from build123d import *

# Parameters (mm, degrees)
ESBO_O1_W                = 174
ESBO_O1_H                = 124
ESBO_O1_R                = 1.5
RESSALTO_EXTRUS_O1_DEPTH = 2
ESBO_O2_R                = 1.3
ESBO_O2_W                = 20
ESBO_O2_H                = 44
ESBO_O2_W_2              = 27
ESBO_O2_H_2              = 11
CORTE_EXTRUS_O1_DEPTH    = 2


with BuildPart() as part:
    # Esboço1 → Ressalto-extrusão1 (new body)
    with BuildSketch(Plane(origin=(0, 0, 0), x_dir=(1, 0, 0), z_dir=(0, 1, 0))):
        Rectangle(ESBO_O1_W, ESBO_O1_H)
        with Locations(Location((-77, 52, 0), (0, 0, 270))):
            Circle(ESBO_O1_R, mode=Mode.SUBTRACT)
        with Locations(Location((-77, -52, 0), (0, 0, 270))):
            Circle(ESBO_O1_R, mode=Mode.SUBTRACT)
        with Locations(Location((77, -52, 0), (0, 0, 270))):
            Circle(ESBO_O1_R, mode=Mode.SUBTRACT)
        with Locations(Location((77, 52, 0), (0, 0, 270))):
            Circle(ESBO_O1_R, mode=Mode.SUBTRACT)
    extrude(amount=RESSALTO_EXTRUS_O1_DEPTH)

    # Esboço2 → Corte-extrusão1 (cut)
    with BuildSketch(Plane(origin=(0, 2, 0), x_dir=(1, 0, 0), z_dir=(0, 1, 0))):
        with Locations(Location((-13.5, -21, 0), (0, 0, 270))):
            Circle(ESBO_O2_R)
        with Locations(Location((-13.5, -29, 0), (0, 0, 270))):
            Circle(ESBO_O2_R)
        with Locations(Location((-13.5, -37, 0), (0, 0, 270))):
            Circle(ESBO_O2_R)
        with Locations(Location((-13.5, -45, 0), (0, 0, 270))):
            Circle(ESBO_O2_R)
        with Locations(Location((13.5, -37, 0), (0, 0, 90))):
            Circle(ESBO_O2_R)
        with Locations(Location((13.5, -45, 0), (0, 0, 90))):
            Circle(ESBO_O2_R)
        with Locations(Location((13.5, -29, 0), (0, 0, 90))):
            Circle(ESBO_O2_R)
        with Locations(Location((13.5, -21, 0), (0, 0, 90))):
            Circle(ESBO_O2_R)
        with Locations((0, -25)):
            Rectangle(ESBO_O2_W, ESBO_O2_H)
        with BuildLine():
            Line((-37, 45), (-37, -45))
            ThreePointArc((-37, -45), (-42, -50), (-47, -45))
            Line((-47, -45), (-47, 45))
            ThreePointArc((-47, 45), (-42, 50), (-37, 45))
        make_face()
        with BuildLine():
            Line((-57, 45), (-57, -45))
            ThreePointArc((-57, -45), (-62, -50), (-67, -45))
            Line((-67, -45), (-67, 45))
            ThreePointArc((-67, 45), (-62, 50), (-57, 45))
        make_face()
        with BuildLine():
            Line((47, 45), (47, -45))
            ThreePointArc((47, -45), (42, -50), (37, -45))
            Line((37, -45), (37, 45))
            ThreePointArc((37, 45), (42, 50), (47, 45))
        make_face()
        with BuildLine():
            Line((67, 45), (67, -45))
            ThreePointArc((67, -45), (62, -50), (57, -45))
            Line((57, -45), (57, 45))
            ThreePointArc((57, 45), (62, 50), (67, 45))
        make_face()
        with BuildLine():
            Line((-20.724176636, 23), (20.724176636, 23))
            ThreePointArc((20.724176636, 23), (25.724176636, 18), (20.724176636, 13))
            Line((20.724176636, 13), (-20.724176636, 13))
            ThreePointArc((-20.724176636, 13), (-25.724176636, 18), (-20.724176636, 23))
        make_face()
        with Locations((0, 46.5)):
            Rectangle(ESBO_O2_W_2, ESBO_O2_H_2)
    extrude(amount=-CORTE_EXTRUS_O1_DEPTH, mode=Mode.SUBTRACT)


solid = part.part
The model under review builds one solid part; all positions refer to its coordinate system, in mm. A direction names the side the tool comes from. Coordinates: 2 decimals unless noted, no trailing zeros. Loops run counter-clockwise (first coordinate to the right, second up) from the corner with the lowest first, then second, coordinate; pieces in that order, holes last. Notation, with made-up numbers: (-26, 32.5) -> (-21, 32.5) arc R36 ccw to (-21, 69.5) -> close; hole circle Ø5 at (-6.75, 78). An arc over 180 degrees is marked (long way). Use a Markdown table: item, result. Add a question column.
1. Draft analysis for pull direction X (two halves, no side actions). For faces 3 (the face through (62, 1, 50)), 4 (the face through (-1, 2, -1)), 5 (the face through (42, 1, -50)), state which applies: pulls with the +X half, pulls with the -X half, needs draft (parallel to the pull), parting line crosses it, or undercut.
2. Add section C-C on z = 41. Write out the cut boundary in (x, y), plus the area to 3 significant figures.
3. Add section B-B on x = 1. Write out the cut boundary in (y, z).
4. Add section A-A on z = -33. Write out the cut boundary in (x, y), plus the area to 3 significant figures.
5. Machinability: for faces 1 (the face through (-1, 0, -1)), 2 (the face through (42, 1, 50)), which of the approach directions +Z, -Z, +X, -X, +Y, -Y give a long, thin tool a straight path to every point of the face, cutting with its end or side? Answer none if there is none.
6. Add section D-D on x = 39.5. Write out the cut boundary in (y, z).
7. To check wall thickness, follow line 1 (X direction, y = 1.2, z = -25); line 2 (Z direction, x = 5, y = 0.5); line 3 (X direction, y = 0.5, z = 52). State the ranges of each line that lie inside material, in increasing order.
Returned:
| question | item | result |
|---|---|---|
| 1 | face 3 | undercut |
| 1 | face 4 | needs draft |
| 1 | face 5 | undercut |
| 2 | outline | (-87, 0) -> (-67, 0) -> (-67, 2) -> (-87, 2) -> close; (-57, 0) -> (-47, 0) -> (-47, 2) -> (-57, 2) -> close; (-37, 0) -> (-10, 0) -> (-10, 2) -> (-37, 2) -> close; (10, 0) -> (37, 0) -> (37, 2) -> (10, 2) -> close; (47, 0) -> (57, 0) -> (57, 2) -> (47, 2) -> close; (67, 0) -> (87, 0) -> (87, 2) -> (67, 2) -> close |
| 2 | area | 228 mm² |
| 3 | outline | (0, -62) -> (2, -62) -> (2, -52) -> (0, -52) -> close; (0, -41) -> (2, -41) -> (2, -23) -> (0, -23) -> close; (0, -13) -> (2, -13) -> (2, 3) -> (0, 3) -> close; (0, 47) -> (2, 47) -> (2, 62) -> (0, 62) -> close |
| 4 | outline | (-87, 0) -> (-67, 0) -> (-67, 2) -> (-87, 2) -> close; (-57, 0) -> (-47, 0) -> (-47, 2) -> (-57, 2) -> close; (-37, 0) -> (37, 0) -> (37, 2) -> (-37, 2) -> close; (47, 0) -> (57, 0) -> (57, 2) -> (47, 2) -> close; (67, 0) -> (87, 0) -> (87, 2) -> (67, 2) -> close |
| 4 | area | 268 mm² |
| 5 | face 1 | +Z, -Z, +X, -X, -Y |
| 5 | face 2 | +Y, -Y |
| 6 | outline | (0, -62) -> (2, -62) -> (2, -49.33) -> (0, -49.33) -> close; (0, 49.33) -> (2, 49.33) -> (2, 62) -> (0, 62) -> close |
| 7 | line 1 | x = -87 to -67, -57 to -47, -37 to 37, 47 to 57, 67 to 87 |
| 7 | line 2 | z = -62 to -52, -41 to -23, -13 to 3, 47 to 62 |
| 7 | line 3 | x = -87 to -78.5, -75.5 to 75.5, 78.5 to 87 |
